```python
from build123d import *

# Parameters (mm, degrees)
BOSS_EXTRUDE1_DEPTH = 10.16
BOSS_EXTRUDE2_DEPTH = 10.16
SKETCH4_W           = 39.941338686
SKETCH4_H           = 10.470779812
BOSS_EXTRUDE3_DEPTH = 5.08
SKETCH6_W           = 10.16
SKETCH6_H           = 55.829783289
BOSS_EXTRUDE5_DEPTH = 5.08
SKETCH9_W           = 10.16
SKETCH9_H           = 6.478239632
BOSS_EXTRUDE6_DEPTH = 34.036
SKETCH12_W          = 45.021338686
SKETCH12_H          = 3.055969703
BOSS_EXTRUDE7_DEPTH = 10.16
SKETCH13_W          = 10.16
SKETCH13_H          = 3.055969703
BOSS_EXTRUDE8_DEPTH = 33.528
SKETCH16_W          = 2.870015597
SKETCH16_H          = 24.680607417
BOSS_EXTRUDE9_DEPTH = 21.13915


with BuildPart() as part:
    # Sketch2 → Boss-Extrude1 (new body)
    with BuildSketch(Plane(origin=(0, 0, 0), x_dir=(0, 0, -1), z_dir=(1, 0, 0))):
        Polygon((0, 14.591559623), (-12.636661314, 7.295779811), (-12.636661314, -7.295779811), (0, -14.591559623), (12.636661314, -7.295779811), (12.636661314, 7.295779811), align=None)
        Polygon((0, 8.241559623), (-7.1374, 4.120779811), (-7.1374, -4.120779811), (0, -8.241559623), (7.1374, -4.120779811), (7.1374, 4.120779811), align=None, mode=Mode.SUBTRACT)
    extrude(amount=BOSS_EXTRUDE1_DEPTH)

    # Sketch3 → Boss-Extrude2 (add)
    with BuildSketch(Plane(origin=(0, 0, 0), x_dir=(0, 0, -1), z_dir=(1, 0, 0))):
        Polygon((12.636661314, -7.295779811), (52.578, -7.295779811), (52.578, 14.591559623), (0, 14.591559623), (12.636661314, 7.295779811), align=None)
    extrude(amount=BOSS_EXTRUDE2_DEPTH)

    # Sketch4 → Boss-Extrude3 (add)
    with BuildSketch(Plane.ZY):
        with Locations((-32.607330657, 9.356169717)):
            Rectangle(SKETCH4_W, SKETCH4_H)
    extrude(amount=BOSS_EXTRUDE3_DEPTH)

    # Sketch6 → Boss-Extrude5 (add)
    with BuildSketch(Plane(origin=(0, 0, -52.578), x_dir=(-1, 0, 0), z_dir=(0, 0, -1))):
        with Locations((-5.08, -13.323332022)):
            Rectangle(SKETCH6_W, SKETCH6_H)
    extrude(amount=BOSS_EXTRUDE5_DEPTH)

    # Sketch9 → Boss-Extrude6 (add)
    with BuildSketch(Plane(origin=(0, -7.295779811, 0), x_dir=(-1, 0, 0), z_dir=(0, -1, 0))):
        with Locations((-5.08, 15.87578113)):
            Rectangle(SKETCH9_W, SKETCH9_H)
    extrude(amount=BOSS_EXTRUDE6_DEPTH)

    # Sketch12 → Boss-Extrude7 (add)
    with BuildSketch(Plane.ZY):
        with Locations((-35.147330657, -39.710238815)):
            Rectangle(SKETCH12_W, SKETCH12_H)
    extrude(amount=BOSS_EXTRUDE7_DEPTH)

    # Sketch13 → Boss-Extrude8 (add)
    with BuildSketch(Plane.XY.offset(-52.578)):
        with Locations((5.08, -39.710238815)):
            Rectangle(SKETCH13_W, SKETCH13_H)
    extrude(amount=BOSS_EXTRUDE8_DEPTH)

    # Sketch16 → Boss-Extrude9 (add)
    with BuildSketch(Plane.ZY):
        with Locations((-56.222992202, -12.340303709)):
            Rectangle(SKETCH16_W, SKETCH16_H)
    extrude(amount=BOSS_EXTRUDE9_DEPTH)


solid = part.part
```
Geometry: final body of the model. Coordinates: model frame, mm. A direction names the side the tool comes from. Round coordinates to 2 decimals unless told otherwise and drop trailing zeros. Order: outer loops, then holes, each group sorted by start corner. A loop starts at its lowest first (then second) coordinate and runs counter-clockwise, first axis right, second up. Notation, with made-up numbers: (88, 54.5) - (96, 54.5) arc R27 cw to (96, 85.5) - close; hole circle Ø7 at (-33, 72.5). An arc over 180 degrees is marked (long way). Use CSV: the item, a comma, the result in double quotes. Start each with the question number.
Q1. Access query for faces 1 (the face through (-3, 9, -12.637)), 2 (the face through (5.009, -10.995, -6.23)), 3 (the face through (-10, -24.681, -56)), 4 (the face through (5.01, 6.15, -3.62)), 5 (the face through (0, -38.182, -35)). Directions: +Z, -Z, +X, -X, +Y, -Y. A direction counts if a zero-diameter tool reaches every point of the face in a straight line with its end or side. Return the directions, or none.
Q2. Material intervals for line 1 along Y through (x, z) = (5.5, -51); line 2 along Y through (x, z) = (-4.5, -28.5); line 3 along Z through (x, y) = (-20, -1.5), sorted ascending. Write a range as from..to.
Q3. Section query A-A (y = -26.5). Return loops of the section in (x, z).
Q4. Mould query, pull axis Z, two halves, no side actions, for faces 6 (the face through (-3, 9, -52.578)), 7 (the face through (5, -23, -19.115)), 8 (the face through (-10, -13, -54.788)). Classes: +Z half, -Z half, draft (parallel to the pull), parting line (faces both ways), or undercut.
Q5. Section query C-C (z = -25). Return loops of the section in (x, y), and give its area (3 significant figures).
Q6. Section query B-B (x = -3.5). Return loops of the section in (y, z), and give its area (3 significant figures).
Q7. Section query D-D (x = 6). Return loops of the section in (y, z), and give its area (3 significant figures).
Q8. First-contact query: pin 1 (5.5 mm diameter, centred on x = -3.5, y = 11.5, fed in from +Z); pin 2 (4 mm diameter, centred on y = -34, z = -20.5, fed in from -X); pin 3 (8 mm diameter, centred on x = 5, y = -17, fed in from +Z). Flat tips, straight axial feed; report the tip coordinate or a pass-through.
Result set:
1,face 1,"+Z, -X, +Y, -Y"
1,face 2,"+X, -X, -Y"
1,face 3,"+Z, -Z, -X"
1,face 4,"+X, -X"
1,face 5,"-X"
2,line 1,"y = -41.24..-38.18, -7.3..14.59"
2,line 2,"y = -41.24..-38.18, 4.12..14.59"
2,line 3,"z = -57.66..-54.79"
3,outline,"(0, -57.66) - (10.16, -57.66) - (10.16, -52.58) - (0, -52.58) - close; (0, -19.11) - (10.16, -19.11) - (10.16, -12.64) - (0, -12.64) - close"
4,face 6,"-Z half"
4,face 7,"undercut"
4,face 8,"+Z half"
5,outline,"(-10.16, -41.24) - (10.16, -41.24) - (10.16, -38.18) - (-10.16, -38.18) - close; (-5.08, 4.12) - (0, 4.12) - (0, -7.3) - (10.16, -7.3) - (10.16, 14.59) - (-5.08, 14.59) - close"
5,area,"338 mm2"
6,outline,"(-41.24, -57.66) - (-38.18, -57.66) - (-38.18, -12.64) - (-41.24, -12.64) - close; (-24.68, -57.66) - (0, -57.66) - (0, -54.79) - (-24.68, -54.79) - close; (4.12, -52.58) - (14.59, -52.58) - (14.59, -12.64) - (4.12, -12.64) - close"
6,area,"627 mm2"
7,outline,"(-41.33, -19.11) - (-41.24, -19.11) - (-41.24, -57.66) - (14.59, -57.66) - (14.59, 0) - (7.3, 12.64) - (-7.3, 12.64) - (-14.59, 0) - (-7.3, -12.64) - (-41.33, -12.64) - close; hole (-38.18, -52.58) - (-7.3, -52.58) - (-7.3, -19.11) - (-38.18, -19.11) - close; hole (-8.24, 0) - (-4.12, -7.14) - (4.12, -7.14) - (8.24, 0) - (4.12, 7.14) - (-4.12, 7.14) - close"
7,area,"1,900 mm2"
8,pin 1,"stops at z = -12.64"
8,pin 2,"stops at x = 0"
8,pin 3,"stops at z = 2.76"
